Build history of the part. All positions in model axes, mm. Face numbers are marked on the shaded views. A direction names the side the tool comes from. Give positions to 0.01 mm unless a question says otherwise; leave off trailing zeros. Loops run counter-clockwise (first coordinate to the right, second up) from the corner with the lowest first, then second, coordinate; pieces in that order, holes last. Notation, with made-up numbers: (32.5, 13.25) - (75.5, 13.25) arc R23 ccw to (75.5, 23.25) - close; hole circle Ø6 at (79.5, 29). An arc over 180 degrees is marked (long way). Return JSON: item names as keys, results as strings. Group by question number.
1) 3-axis set-ups, long thin cutter, end or side, ignore diameter. For the marked faces 1, 2, 3, 4 and 5: which of +Z, -Z, +X, -X, +Y, -Y reach the whole face in a straight line?
2) Drill centre lines: probe 1 along X at (y, z) = (-18.1, 4); probe 2 along Z at (x, y) = (-12.5, -2); probe 3 along X at (y, z) = (-10, 5.5). Where is each one in solid material? Low to high. Write a range as from..to.
3) Drop flat-ended pins along their axis: pin 1 (0.9 mm diameter, centred on x = 15.5, y = -19, fed in from -Z); pin 2 (4 mm diameter, centred on x = 20, z = 4, fed in from +Y); pin 3 (4 mm diameter, centred on x = 5.5, y = -4.5, fed in from +Z); pin 4 (2 mm diameter, centred on x = 0, y = 3, fed in from -Z). Give the stop position or say it passes through.
4) Mould opens along Y. For the marked faces 6, 7 and 8 say: released by +Y, released by -Y, zero draft, split by the parting line, or undercut.
5) Slice it at C-C (y = 10.5). List the corners of the cut face in (x, z), and give its area (3 significant figures).
6) Slice it at B-B (x = 17). List the corners of the cut face in (y, z).
7) Slice it at D-D (x = 3.5). List the corners of the cut face in (y, z), and give its area (3 significant figures).
8) Slice it at A-A (z = 32). List the corners of the cut face in (x, y), and give its area (3 significant figures).
```python
from build123d import *

# Parameters (mm, degrees)
CROQUIS1_R              = 9.5
SALIENTE_EXTRUIR1_DEPTH = 36
CROQUIS2_W              = 20.1
CROQUIS2_H              = 30
CORTAR_EXTRUIR2_DEPTH   = 49.703182648
CROQUIS3_R              = 9.5
CROQUIS3_R_2            = 6
SALIENTE_EXTRUIR2_DEPTH = 2
SALIENTE_EXTRUIR3_START = -2
CROQUIS4_R              = 9.5
CROQUIS4_R_2            = 6
SALIENTE_EXTRUIR3_DEPTH = 2
SALIENTE_EXTRUIR4_DEPTH = 3
CROQUIS6_R              = 1.5
CORTAR_EXTRUIR3_DEPTH   = 55.415071442
REDONDEO3_R             = 2


with BuildPart() as part:
    # Croquis1 → Saliente-Extruir1 (new body)
    with BuildSketch(Plane.XY):
        with BuildLine():
            Line((-13, 0), (-13, -20))
            Line((-13, -20), (13, -20))
            Line((13, -20), (13, 0))
            ThreePointArc((13, 0), (0, 13), (-13, 0))
        make_face()
        Circle(CROQUIS1_R, mode=Mode.SUBTRACT)
    extrude(amount=SALIENTE_EXTRUIR1_DEPTH)

    # Croquis2 → Cortar-Extruir2 (cut, through all)
    with BuildSketch(Plane(origin=(13, 0, 0), x_dir=(0, 0, -1), z_dir=(1, 0, 0))):
        with Locations((-18, -2)):
            Rectangle(CROQUIS2_W, CROQUIS2_H)
    extrude(amount=-CORTAR_EXTRUIR2_DEPTH, mode=Mode.SUBTRACT)

    # Croquis3 → Saliente-Extruir2 (add)
    with BuildSketch(Plane(origin=(0, 0, 28.05), x_dir=(-1, 0, 0), z_dir=(0, 0, -1))):
        with Locations(Location((0, 0, 0), (0, 0, 90))):
            Circle(CROQUIS3_R)
        with Locations(Location((0, 0, 0), (0, 0, 90))):
            Circle(CROQUIS3_R_2, mode=Mode.SUBTRACT)
    extrude(amount=-SALIENTE_EXTRUIR2_DEPTH)

    # Croquis4 → Saliente-Extruir3 (add)
    with BuildSketch(Plane.XY.offset(7.95).offset(SALIENTE_EXTRUIR3_START)):
        Circle(CROQUIS4_R)
        with Locations(Location((0, 0, 0), (0, 0, 90))):
            Circle(CROQUIS4_R_2, mode=Mode.SUBTRACT)
    extrude(amount=SALIENTE_EXTRUIR3_DEPTH)

    # Croquis5 → Saliente-Extruir4 (add)
    with BuildSketch(Plane.XZ.offset(20)):
        with BuildLine():
            Line((13, 36), (20, 36))
            ThreePointArc((20, 36), (24, 32), (20, 28))
            Line((20, 28), (13, 28))
            Line((13, 28), (13, 36))
        make_face()
        with BuildLine():
            Line((13, 0), (20, 0))
            ThreePointArc((20, 0), (24, 4), (20, 8))
            Line((20, 8), (13, 8))
            Line((13, 8), (13, 0))
        make_face()
        with BuildLine():
            Line((-13, 0), (-20, 0))
            ThreePointArc((-20, 0), (-24, 4), (-20, 8))
            Line((-20, 8), (-13, 8))
            Line((-13, 8), (-13, 0))
        make_face()
        with BuildLine():
            Line((-13, 28), (-13, 36))
            Line((-13, 36), (-20, 36))
            ThreePointArc((-20, 36), (-24, 32), (-20, 28))
            Line((-20, 28), (-13, 28))
        make_face()
    extrude(amount=-SALIENTE_EXTRUIR4_DEPTH)

    # Croquis6 → Cortar-Extruir3 (cut, through all)
    with BuildSketch(Plane.XZ.offset(20)):
        with Locations(Location((-20, 32, 0), (0, 0, 270))):
            Circle(CROQUIS6_R)
        with Locations(Location((20, 32, 0), (0, 0, 270))):
            Circle(CROQUIS6_R)
        with Locations(Location((-20, 4, 0), (0, 0, 270))):
            Circle(CROQUIS6_R)
        with Locations(Location((20, 4, 0), (0, 0, 270))):
            Circle(CROQUIS6_R)
    extrude(amount=-CORTAR_EXTRUIR3_DEPTH, mode=Mode.SUBTRACT)

    # Redondeo3
    redondeo3_edges = [part.edges().sort_by_distance(p)[0] for p in [
        (13, -17, 18),
        (-13, -17, 18),
        (-13, -17, 32.025),
        (-13, -17, 3.975),
        (13, -17, 3.975),
        (13, -17, 32.025),
    ]]
    fillet(redondeo3_edges, radius=REDONDEO3_R)


solid = part.part
```
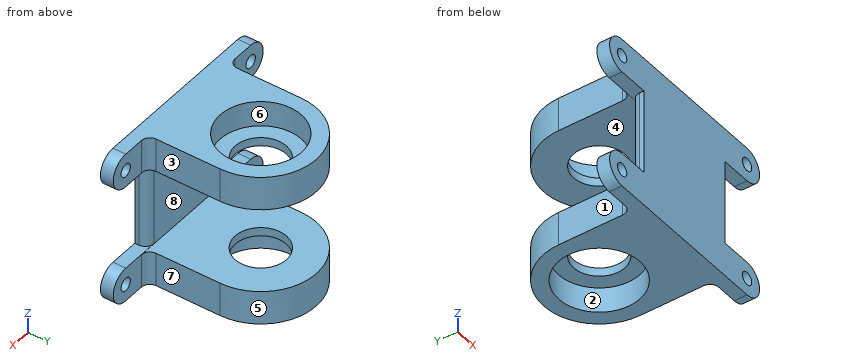
Results:
{
 "1": {"face 1": "+Z, -Z, -X, +Y", "face 2": "-Z", "face 3": "+Z, -Z, +X, +Y", "face 4": "+X, -X, +Y", "face 5": "+Z, -Z, +Y"},
 "2": {"probe 1": "-24..-21.5, -18.5..18.5, 21.5..24", "probe 2": "0..7.95, 28.05..36", "probe 3": "-13..13"},
 "3": {"pin 1": "z = 0", "pin 2": "y = -17", "pin 3": "z = 30.05", "pin 4": "through"},
 "4": {"face 6": "undercut", "face 7": "zero draft", "face 8": "released by +Y"},
 "5": {"outline": "(-7.66, 0) - (7.66, 0) - (7.66, 7.95) - (-7.66, 7.95) - close; (-7.66, 28.05) - (7.66, 28.05) - (7.66, 36) - (-7.66, 36) - close", "area": "244 mm2"},
 "6": {"outline": "(-20, 0) - (-17, 0) - (-17, 8) - (-20, 8) - close; (-20, 28) - (-17, 28) - (-17, 36) - (-20, 36) - close"},
 "7": {"outline": "(-20, 0) - (-8.83, 0) - (-8.83, 5.95) - (-4.87, 5.95) - (-4.87, 7.95) - (-17, 7.95) - (-17, 28.05) - (-4.87, 28.05) - (-4.87, 30.05) - (-8.83, 30.05) - (-8.83, 36) - (-20, 36) - close; (4.87, 5.95) - (8.83, 5.95) - (8.83, 0) - (12.52, 0) - (12.52, 7.95) - (4.87, 7.95) - close; (4.87, 28.05) - (12.52, 28.05) - (12.52, 36) - (8.83, 36) - (8.83, 30.05) - (4.87, 30.05) - close", "area": "328 mm2"},
 "8": {"outline": "(-24, -20) - (-21.5, -20) - (-21.5, -17) - (-24, -17) - close; (-18.5, -20) - (18.5, -20) - (18.5, -17) - (15, -17) arc R2 cw to (13, -15) - (13, 0) arc R13 ccw to (-13, 0) - (-13, -15) arc R2 cw to (-15, -17) - (-18.5, -17) - close; (21.5, -20) - (24, -20) - (24, -17) - (21.5, -17) - close; hole circle Ø19 at (0, 0)", "area": "552 mm2"}
}
